```python
from build123d import *

# Parameters (mm, degrees)
F0_R     = 1.6
F0_R_2   = 4.38006
F1_DEPTH = 2.5
F3_DEPTH = 1
F4_R     = 3
F4_R_2   = 1.6
F5_DEPTH = 1
F7_DEPTH = 2.5
F8_R     = 1.7
F9_DEPTH = 2.501
F10_D    = 4.7


with BuildPart() as f1:
    # F0 (on Top) → F1 (new body)
    with BuildSketch(Plane.XY):
        with BuildLine():
            Line((13.65, 20), (-13.65, 20))
            ThreePointArc((-13.65, 20), (-18.140128, 18.140128), (-20, 13.65))
            Line((-20, 13.65), (-20, -13.65))
            ThreePointArc((-20, -13.65), (-18.140128, -18.140128), (-13.65, -20))
            Line((-13.65, -20), (13.65, -20))
            ThreePointArc((13.65, -20), (18.140128, -18.140128), (20, -13.65))
            Line((20, -13.65), (20, 13.65))
            ThreePointArc((20, 13.65), (18.140128, 18.140128), (13.65, 20))
        make_face()
        with Locations((-16, -16)):
            Circle(F0_R, mode=Mode.SUBTRACT)
        with BuildLine():
            ThreePointArc((-1, -18.723314), (-13.258252, -13.258252), (-18.723314, -1))
            Line((-18.723314, -1), (-13.327216, -1))
            ThreePointArc((-13.327216, -1), (-9.450256, -9.450256), (-1, -13.327216))
            Line((-1, -13.327216), (-1, -18.723314))
        make_face(mode=Mode.SUBTRACT)
        with BuildLine():
            ThreePointArc((-5.873836, -1), (-4.213191, -4.213191), (-1, -5.873836))
            Line((-1, -5.873836), (-1, -11.296782))
            ThreePointArc((-1, -11.296782), (-8.019267, -8.019267), (-11.296782, -1))
            Line((-11.296782, -1), (-5.873836, -1))
        make_face(mode=Mode.SUBTRACT)
        with Locations((16, -16)):
            Circle(F0_R, mode=Mode.SUBTRACT)
        with BuildLine():
            ThreePointArc((18.723314, -1), (13.258252, -13.258252), (1, -18.723314))
            Line((1, -18.723314), (1, -13.327216))
            ThreePointArc((1, -13.327216), (9.450256, -9.450256), (13.327216, -1))
            Line((13.327216, -1), (18.723314, -1))
        make_face(mode=Mode.SUBTRACT)
        with BuildLine():
            ThreePointArc((1, -5.873836), (4.213191, -4.213191), (5.873836, -1))
            Line((5.873836, -1), (11.296782, -1))
            ThreePointArc((11.296782, -1), (8.019267, -8.019267), (1, -11.296782))
            Line((1, -11.296782), (1, -5.873836))
        make_face(mode=Mode.SUBTRACT)
        with BuildLine():
            ThreePointArc((-11.296782, 1), (-8.019267, 8.019267), (-1, 11.296782))
            Line((-1, 11.296782), (-1, 5.873836))
            ThreePointArc((-1, 5.873836), (-4.213191, 4.213191), (-5.873836, 1))
            Line((-5.873836, 1), (-11.296782, 1))
        make_face(mode=Mode.SUBTRACT)
        with BuildLine():
            ThreePointArc((-18.723314, 1), (-13.258252, 13.258252), (-1, 18.723314))
            Line((-1, 18.723314), (-1, 13.327216))
            ThreePointArc((-1, 13.327216), (-9.450256, 9.450256), (-13.327216, 1))
            Line((-13.327216, 1), (-18.723314, 1))
        make_face(mode=Mode.SUBTRACT)
        with Locations((-16, 16)):
            Circle(F0_R, mode=Mode.SUBTRACT)
        Circle(F0_R_2, mode=Mode.SUBTRACT)
        with BuildLine():
            Line((11.296782, 1), (5.873836, 1))
            ThreePointArc((5.873836, 1), (4.213191, 4.213191), (1, 5.873836))
            Line((1, 5.873836), (1, 11.296782))
            ThreePointArc((1, 11.296782), (8.019267, 8.019267), (11.296782, 1))
        make_face(mode=Mode.SUBTRACT)
        with BuildLine():
            Line((1, 13.327216), (1, 18.723314))
            ThreePointArc((1, 18.723314), (13.258252, 13.258252), (18.723314, 1))
            Line((18.723314, 1), (13.327216, 1))
            ThreePointArc((13.327216, 1), (9.450256, 9.450256), (1, 13.327216))
        make_face(mode=Mode.SUBTRACT)
        with Locations((16, 16)):
            Circle(F0_R, mode=Mode.SUBTRACT)
    extrude(amount=F1_DEPTH)

    # F2 (on face) → F3 (cut)
    with BuildSketch(Plane.XY.offset(2.5)):
        with BuildLine():
            ThreePointArc((18.75, 0), (12.899855, 13.607213), (-1, 18.723314))
            ThreePointArc((-1, 18.723314), (-13.258252, 13.258252), (-18.723314, 1))
            ThreePointArc((-18.723314, 1), (-18.75, 0), (-18.723314, -1))
            ThreePointArc((-18.723314, -1), (-13.258252, -13.258252), (-1, -18.723314))
            ThreePointArc((-1, -18.723314), (12.899855, -13.607213), (18.75, 0))
        make_face()
    extrude(amount=-F3_DEPTH, mode=Mode.SUBTRACT)

    # F4 (on face) → F5 (cut)
    with BuildSketch(Plane(origin=(0, 0, 0), x_dir=(1, 0, 0), z_dir=(0, 0, -1))):
        with Locations((-16, 16)):
            Circle(F4_R)
        with Locations((-16, 16)):
            Circle(F4_R_2, mode=Mode.SUBTRACT)
        with Locations((16, 16)):
            Circle(F4_R)
        with Locations((16, 16)):
            Circle(F4_R_2, mode=Mode.SUBTRACT)
        with Locations((16, -16)):
            Circle(F4_R)
        with Locations((16, -16)):
            Circle(F4_R_2, mode=Mode.SUBTRACT)
        with Locations((-16, -16)):
            Circle(F4_R)
        with Locations((-16, -16)):
            Circle(F4_R_2, mode=Mode.SUBTRACT)
    extrude(amount=-F5_DEPTH, mode=Mode.SUBTRACT)

    # F6 (on face) → F7 (join, through all)
    with BuildSketch(Plane(origin=(0, 0, 0), x_dir=(1, 0, 0), z_dir=(0, 0, -1))):
        with BuildLine():
            ThreePointArc((-13.65, 21.27), (-19.038154, 19.038154), (-21.27, 13.65))
            Line((-21.27, 13.65), (-21.27, -13.65))
            ThreePointArc((-21.27, -13.65), (-19.038154, -19.038154), (-13.65, -21.27))
            Line((-13.65, -21.27), (13.65, -21.27))
            ThreePointArc((13.65, -21.27), (19.038154, -19.038154), (21.27, -13.65))
            Line((21.27, -13.65), (21.27, 13.65))
            ThreePointArc((21.27, 13.65), (19.038154, 19.038154), (13.65, 21.27))
            Line((13.65, 21.27), (-13.65, 21.27))
        make_face()
        with BuildLine():
            ThreePointArc((-20, 13.65), (-18.140128, 18.140128), (-13.65, 20))
            Line((-13.65, 20), (13.65, 20))
            ThreePointArc((13.65, 20), (18.140128, 18.140128), (20, 13.65))
            Line((20, 13.65), (20, -13.65))
            ThreePointArc((20, -13.65), (18.140128, -18.140128), (13.65, -20))
            Line((13.65, -20), (-13.65, -20))
            ThreePointArc((-13.65, -20), (-18.140128, -18.140128), (-20, -13.65))
            Line((-20, -13.65), (-20, 13.65))
        make_face(mode=Mode.SUBTRACT)
    extrude(amount=-F7_DEPTH)

    # F8 (on face) → F9 (cut, through all)
    with BuildSketch(Plane.XY.offset(2.5)):
        with Locations((16, 16)):
            Circle(F8_R)
        with Locations((16, -16)):
            Circle(F8_R)
        with Locations((-16, -16)):
            Circle(F8_R)
        with Locations((-16, 16)):
            Circle(F8_R)
    extrude(amount=-F9_DEPTH, mode=Mode.SUBTRACT)

    # F10 (through all)
    with Locations(Plane(origin=(0, 0, 0), x_dir=(1, 0, 0), z_dir=(0, 0, -1))):
        with Locations((-16, -16), (16, -16), (16, 16), (-16, 16)):
            Hole(F10_D / 2)


solid = f1.part
```
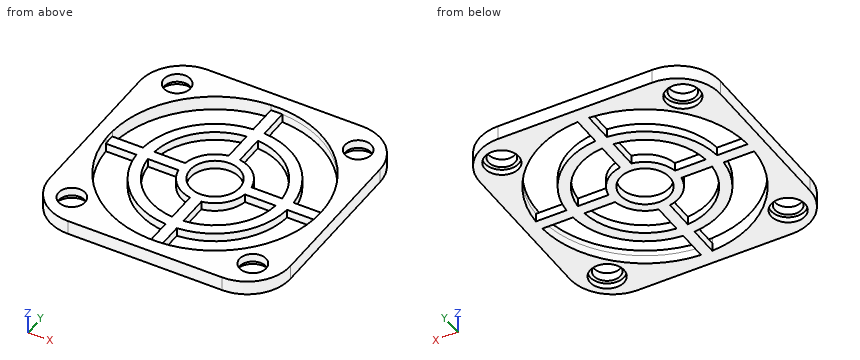
The model under review builds one solid part; all positions refer to its coordinate system, in mm. Round coordinates to 2 decimals unless told otherwise and drop trailing zeros. Order: outer loops, then holes, each group sorted by start corner. A loop starts at its lowest first (then second) coordinate and runs counter-clockwise, first axis right, second up.
Item 1: Add section B-B, the plane x = 0. State the section outline as (y, z) points, and give its area (3 significant figures).
Working result:
outline: (-21.27, 0) - (-4.38, 0) - (-4.38, 1.5) - (-18.75, 1.5) - (-18.75, 2.5) - (-21.27, 2.5) - close; (4.38, 0) - (21.27, 0) - (21.27, 2.5) - (18.75, 2.5) - (18.75, 1.5) - (4.38, 1.5) - close
area: 55.7 mm2
Item 2: Add section C-C, the plane x = 16. State the section outline as (y, z) points.
Working result:
outline: (-20.9, 0) - (-19, 0) - (-19, 1) - (-18.35, 1) - (-18.35, 2.5) - (-20.9, 2.5) - close; (-13.65, 1) - (-13, 1) - (-13, 0) - (-9.78, 0) - (-9.78, 2.5) - (-13.65, 2.5) - close; (-1, 0) - (1, 0) - (1, 1.5) - (-1, 1.5) - close; (9.78, 0) - (13, 0) - (13, 1) - (13.65, 1) - (13.65, 2.5) - (9.78, 2.5) - close; (18.35, 1) - (19, 1) - (19, 0) - (20.9, 0) - (20.9, 2.5) - (18.35, 2.5) - close
Item 3: For pin 1 (1.2 mm diameter, centred on x = -15.5, z = 0.5, fed in from -Y); pin 2 (5.5 mm diameter, centred on x = -16, y = -16, fed in from -Z); pin 3 (18.5 mm diameter, centred on x = -8.5, y = 2.5, fed in from +Z); pin 4 (1.8 mm diameter, centred on x = -17, y = -16, fed in from -Z), all flat-tipped, find the tip position at first contact; note any pin that passes through.
Working result:
pin 1: stops at y = -21.17
pin 2: stops at z = 1
pin 3: stops at z = 1.5
pin 4: passes through
Item 4: Add section A-A, the plane z = 1.95. State the section outline as (x, y) points.
Working result:
outline: (-21.27, -13.65) arc R7.62 ccw to (-13.65, -21.27) - (13.65, -21.27) arc R7.62 ccw to (21.27, -13.65) - (21.27, 13.65) arc R7.62 ccw to (13.65, 21.27) - (-13.65, 21.27) arc R7.62 ccw to (-21.27, 13.65) - close; hole (-18.72, -1) arc R18.75 ccw to (-1, -18.72) arc R18.75 ccw to (18.75, 0) arc R18.75 ccw to (-1, 18.72) arc R18.75 ccw to (-18.72, 1) arc R18.75 ccw to start; hole circle Ø4.7 at (-16, -16); hole circle Ø4.7 at (-16, 16); hole circle Ø4.7 at (16, -16); hole circle Ø4.7 at (16, 16)
Item 5: Add section D-D, the plane y = -8.5. State the section outline as (x, z) points.
Working result:
outline: (-21.27, 0) - (-16.71, 0) - (-16.71, 2.5) - (-21.27, 2.5) - close; (-10.31, 0) - (-7.51, 0) - (-7.51, 1.5) - (-10.31, 1.5) - close; (-1, 0) - (1, 0) - (1, 1.5) - (-1, 1.5) - close; (7.51, 0) - (10.31, 0) - (10.31, 1.5) - (7.51, 1.5) - close; (16.71, 0) - (21.27, 0) - (21.27, 2.5) - (16.71, 2.5) - close
Item 6: To check wall thickness, follow probe 1 along X at (y, z) = (-16, 1.4); probe 2 along Y at (x, z) = (16, 2.1); probe 3 along Y at (x, z) = (5, 1.05). State the ranges of each line that lie inside material, in increasing order.
Working result:
probe 1: x = -20.9 to -18.35, -13.65 to -9.78, -1 to 1, 9.78 to 13.65, 18.35 to 20.9
probe 2: y = -20.9 to -18.35, -13.65 to -9.78, 9.78 to 13.65, 18.35 to 20.9
probe 3: y = -21.27 to -18.07, -12.39 to -10.18, -3.24 to 3.24, 10.18 to 12.39, 18.07 to 21.27
